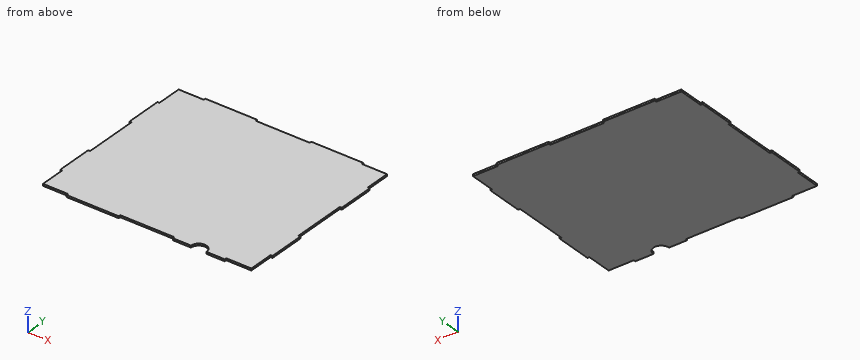
from build123d import *

# Parameters (mm, degrees)
F0_W     = 348.615
F0_H     = 297.815
F1_DEPTH = 3.175
F2_W     = 44.45
F2_H     = 3.175
F2_W_2   = 3.175
F2_H_2   = 44.45
F3_DEPTH = 3.176
F5_DEPTH = 3.176


with BuildPart() as f1:
    # F0 (on Top) → F1 (new body)
    with BuildSketch(Plane.XY):
        Rectangle(F0_W, F0_H)
    extrude(amount=F1_DEPTH)

    # F2 (on face) → F3 (cut, through all)
    with BuildSketch(Plane.XY.offset(3.175)):
        Polygon((-129.8575, 145.7325), (-129.8575, 148.9075), (-174.3075, 148.9075), (-174.3075, 104.4575), (-171.1325, 104.4575), (-171.1325, 145.7325), align=None)
        with Locations((-22.225, 147.32)):
            Rectangle(F2_W, F2_H)
        with Locations((22.225, 147.32)):
            Rectangle(F2_W, F2_H)
        with Locations((-172.72, 22.225)):
            Rectangle(F2_W_2, F2_H_2)
        with Locations((-172.72, -22.225)):
            Rectangle(F2_W_2, F2_H_2)
        with Locations((172.72, -22.225)):
            Rectangle(F2_W_2, F2_H_2)
        with Locations((172.72, 22.225)):
            Rectangle(F2_W_2, F2_H_2)
        Polygon((171.1325, 145.7325), (171.1325, 104.4575), (174.3075, 104.4575), (174.3075, 148.9075), (129.8575, 148.9075), (129.8575, 145.7325), align=None)
        with Locations((-22.225, -147.32)):
            Rectangle(F2_W, F2_H)
        with Locations((22.225, -147.32)):
            Rectangle(F2_W, F2_H)
        Polygon((-171.1325, -145.7325), (-171.1325, -104.4575), (-174.3075, -104.4575), (-174.3075, -148.9075), (-129.8575, -148.9075), (-129.8575, -145.7325), align=None)
        Polygon((129.8575, -145.7325), (129.8575, -148.9075), (174.3075, -148.9075), (174.3075, -104.4575), (171.1325, -104.4575), (171.1325, -145.7325), align=None)
    extrude(amount=-F3_DEPTH, mode=Mode.SUBTRACT)

    # F4 (on face) → F5 (cut, through all)
    with BuildSketch(Plane.XY.offset(3.175)):
        with BuildLine():
            Line((74.45375, -148.9075), (99.85375, -148.9075))
            ThreePointArc((99.85375, -148.9075), (87.15375, -136.2075), (74.45375, -148.9075))
        make_face()
    extrude(amount=-F5_DEPTH, mode=Mode.SUBTRACT)


solid = f1.part
Model file for the job. Use its own axes, mm. Coordinates: 2 decimals unless noted, no trailing zeros. Loops run counter-clockwise (first coordinate to the right, second up) from the corner with the lowest first, then second, coordinate; pieces in that order, holes last. Notation, with made-up numbers: (38, 4) -> (72, 4) arc R23 ccw to (72, 43) -> close; hole circle Ø4 at (-29.5, 48.25). An arc over 180 degrees is marked (long way). Use one line per item in the form item = value. Start each with the question number.
(1) Cut at A-A on y = -5.5. Give the cut face in (x, z) (1 decimal), and give its area (3 significant figures).
(2) Probe probe 1 along X at (y, z) = (-43.5, 0.8); probe 2 along Y at (x, z) = (157, 1.75); probe 3 along Y at (x, z) = (82, 0.65). List the from-to ranges inside material, lowest first. Write a range as from..to.
(3) Cut at B-B on x = 18. Give the cut face in (y, z) (1 decimal), and give its area (3 significant figures).
(4) Flat gauge pins, fed straight in: pin 1 (1 mm diameter, centred on x = 12.5, z = 2.5, fed in from +Y); pin 2 (1 mm diameter, centred on x = -172, z = 1.5, fed in from -Y); pin 3 (1.5 mm diameter, centred on y = 40, z = 1, fed in from -X). Where does each tip first touch, or does it go through?
Values:
q1.outline = (-171.1, 0) -> (171.1, 0) -> (171.1, 3.2) -> (-171.1, 3.2) -> close
q1.area = 1,090 mm2
q2.probe_1 = -171.13..171.13
q2.probe_2 = -145.73..145.73
q2.probe_3 = -137.3..148.91
q3.outline = (-145.7, 0) -> (145.7, 0) -> (145.7, 3.2) -> (-145.7, 3.2) -> close
q3.area = 925 mm2
q4.pin_1 = 145.73
q4.pin_2 = -104.46
q4.pin_3 = -171.13
